Source: CAD feature listing. Evaluate the final solid. Frame: model axes, mm. A direction names the side the tool comes from. Coordinates: 2 decimals unless noted, no trailing zeros. Write each loop counter-clockwise with the first axis right and the second up, starting at its lowest first coordinate (ties: lowest second). Pieces come first, ordered by that corner, then holes. Notation, with made-up numbers: (11.5, -30) - (58.5, -30) arc R29 cw to (58.5, 6) - close; hole circle Ø3 at (76, 82). An arc over 180 degrees is marked (long way). One line per question, with ' | ' between items. Start each with the question number.
Q1. Line query: line 1 (Z direction, x = 76, y = 2.3); line 2 (Z direction, x = 76, y = 0.8); line 3 (X direction, y = 2.45, z = 30). Output: solid intervals per line, ascending.
Q2. Cut plane B-B, the plane x = 16. Return loops of the section in (y, z), plus the area to 3 significant figures.
Q3. Contact query for flat-ended pins moving along their axis: P1, Ø1.5, axis at y = 2, z = -9, coming from the +X side; P2, Ø4, axis at x = 76, z = -30, coming from the -Y side; P3, Ø0.9, axis at x = 91.5, y = 1, coming from the -Z side. Output: stop coordinate, or through.
Q4. Cut plane C-C, the plane x = -44. Return loops of the section in (y, z), plus the area to 3 significant figures.
Q5. Cut plane A-A, the plane z = 0. Return loops of the section in (x, y), plus the area to 3 significant figures.
Q6. Cut plane D-D, the plane y = 2.35. Give the number of separate pieces and of enclosed holes in the cut face, plus the area to 3 significant figures.
Q7. Access query for faces 5 (the face through (-58.8, 2, 20)), 6 (the face through (90.641, 1.479, 41.203)), 7 (the face through (96.07, 1.48, 53.5)). Directions: +Z, -Z, +X, -X, +Y, -Y. A direction counts if a zero-diameter tool reaches every point of the face in a straight line with its end or side. Return the directions, or none.
Q8. Draft query along X for faces 1 (the face through (52.95, 1.52, 15.32)), 2 (the face through (-65.5, 2, -27)), 3 (the face through (-44.208, 2.31, -31.586)), 4 (the face through (90.703, 1.479, 47.859)). Return one class per face: +X half, -X half, draft (parallel to the pull), parting line (faces both ways), or undercut.
Autodesk Inventor part; units mm, degrees
ref_plane "YZ Plane" through (0, 0, 0) normal (1, 0, 0) x (0, 1, 0)
ref_plane "XZ Plane" through (0, 0, 0) normal (0, 1, 0) x (-1, 0, 0)
ref_plane "XY Plane" through (0, 0, 0) normal (0, 0, 1) x (1, 0, 0)
sketch "Sketch1" plane through (0, 0, 0) normal (0, 1, 0) x (-1, 0, 0)
  circle A0 centre (0, 0) radius 40
  circle A1 centre (0, 0) radius 25
  dimension "d1" = 50
  dimension "d13" = 15
extrude "Extrusion1" add sketch "Sketch1" along normal blind 5
sketch "Sketch2" plane through (0, 5, 0) normal (0, 1, 0) x (1, 0, 0)
  circle A0 centre (-33, 0) radius 1.25
  circle A1 centre (0, 0) radius 25
  circle A2 centre (0, 0) radius 33 construction
  dimension "d4" = 2.5
  dimension "d12" = 8
extrude "Extrusion2" cut sketch "Sketch2" against normal blind 10 contours A0
pattern_circular "Circular Pattern1" count 6 over 360 about axis through (0, 0, 0) along (0, 1, 0) of "Extrusion2"
sketch "Sketch3" plane through (0, 5, 0) normal (0, 1, 0) x (1, 0, 0)
  line L0 (-85, -42.5) -> (85, -42.5)
  line L1 (85, -42.5) -> (85, 42.5)
  line L2 (85, 42.5) -> (-85, 42.5)
  line L3 (-85, 42.5) -> (-85, -42.5)
  line L4 (-85, -42.5) -> (85, 42.5) construction
  line L5 (85, -42.5) -> (-85, 42.5) construction
  line L6 (34.5, 15.5) -> (65.5, 15.5) construction
  line L7 (65.5, 15.5) -> (65.5, -15.5) construction
  line L8 (65.5, -15.5) -> (34.5, -15.5) construction
  line L9 (34.5, -15.5) -> (34.5, 15.5) construction
  line L10 (34.5, 15.5) -> (65.5, -15.5) construction
  line L11 (65.5, 15.5) -> (34.5, -15.5) construction
  circle A0 centre (34.5, 15.5) radius 1.5
  circle A1 centre (65.5, 15.5) radius 1.5
  circle A2 centre (65.5, -15.5) radius 1.5
  circle A3 centre (34.5, -15.5) radius 1.5
  line L12 (0, 0) -> (50, 0) construction
  circle A4 centre (0, 0) radius 40
  circle A5 centre (0, 0) radius 40
  line L13 (-50, 42.5) -> (-50, -42.5)
  circle A6 centre (50, 0) radius 12
  dimension "d14" = 85
  dimension "d15" = 170
  dimension "d16" = 31
  dimension "d17" = 31
  dimension "d18" = 3
  dimension "d19" = 3
  dimension "d20" = 3
  dimension "d21" = 3
  dimension "d22" = 50
  dimension "d23" = 35
  dimension "d26" = 24
extrude "Extrusion3" add sketch "Sketch3" against normal blind 5 contours L13 L2 L1 L0
sketch "Sketch4" plane through (0, 5, 0) normal (0, 1, 0) x (1, 0, 0)
  arc A0 (39.56, -5.9166) -> (39.56, 5.9166) centre (50, 0) ccw
  circle A1 centre (50, 0) radius 12
  point P0 (0, 0)
  point P1 (39.56, 5.9166)
  point P2 (39.56, -5.9166)
extrude "Extrusion4" cut sketch "Sketch4" against normal blind 5
sketch "Sketch5" plane through (0, 5, 0) normal (0, 1, 0) x (1, 0, 0)
  circle A0 centre (65.5, 15.5) radius 1.5
  circle A1 centre (65.5, 15.5) radius 1.5
  line L0 (34.5, -15.5) -> (65.5, -15.5)
  line L1 (65.5, -15.5) -> (65.5, 15.5)
  line L2 (65.5, 15.5) -> (34.5, 15.5)
  line L3 (34.5, 15.5) -> (34.5, -15.5)
  circle A2 centre (50, 0) radius 12
  line L4 (34.5, -15.5) -> (65.5, 15.5) construction
  line L5 (65.5, -15.5) -> (34.5, 15.5) construction
  circle A3 centre (34.5, 15.5) radius 1.5
  circle A4 centre (34.5, -15.5) radius 1.5
  point P0 (0, 0)
  dimension "d30" = 3
  dimension "d31" = 3
extrude "Extrusion5" cut sketch "Sketch5" against normal blind 5 contours A3 L3 L2 | L2 L3 A3 | A4 L3 L0 | L0 L3 A4
sketch "Sketch6" plane through (0, 5, 0) normal (0, 1, 0) x (1, 0, 0)
  line L0 (-65.5, -55) -> (97.5, -55)
  line L1 (97.5, -55) -> (97.5, 55)
  line L2 (97.5, 55) -> (-65.5, 55)
  line L3 (-65.5, 55) -> (-65.5, -55)
  line L4 (-65.5, -55) -> (97.5, 55) construction
  line L5 (97.5, -55) -> (-65.5, 55) construction
  line L6 (-65.5, 4) -> (-58.8, 4)
  line L7 (-58.8, 4) -> (-58.8, -55)
  line L8 (-58.8, -55) -> (-65.5, -55)
  line L9 (-65.5, -55) -> (-65.5, 4)
  line L10 (97.5, 55) -> (90.8, 55)
  line L11 (90.8, 55) -> (90.8, -4)
  line L12 (90.8, -4) -> (97.5, -4)
  line L13 (97.5, -4) -> (97.5, 55)
  line L14 (-50, -42.5) -> (-50, 42.5)
  line L15 (85, 42.5) -> (85, -42.5)
  line L16 (-50, 42.5) -> (85, 42.5)
  line L17 (85, 42.5) -> (85, -42.5)
  line L18 (85, -42.5) -> (-50, -42.5)
  line L19 (-50, -42.5) -> (-50, 42.5)
  point P0 (0, 0)
  point P1 (16, 0)
  dimension "d34" = 16
  dimension "d35" = 110
  dimension "d36" = 163
  dimension "d37" = 6.7
  dimension "d38" = 6.7
  dimension "d40" = 51
  dimension "d41" = 51
extrude "Extrusion6" add sketch "Sketch6" against normal blind 5 contours L7 L6 L3 L2 L11 L12 L1 L0
sketch "Sketch7" plane through (0, 5, 0) normal (0, 1, 0) x (1, 0, 0)
  line L0 (97.5, -49) -> (89.5, -49)
  line L1 (89.5, -49) -> (89.5, -40)
  line L2 (89.5, -40) -> (97.5, -40)
  line L3 (97.5, -40) -> (97.5, -49)
  line L4 (-58.8, -55) -> (97.5, -55)
  line L5 (97.5, -55) -> (97.5, -4)
  line L6 (97.5, -28) -> (93.5, -28)
  line L7 (93.5, -28) -> (93.5, -32)
  line L8 (93.5, -32) -> (97.5, -32)
  line L9 (97.5, -32) -> (97.5, -28)
  point P0 (0, 0)
  dimension "d44" = 6
  dimension "d45" = 9
  dimension "d46" = 8
  dimension "d47" = 8
  dimension "d48" = 4
  dimension "d49" = 4
extrude "Extrusion7" cut sketch "Sketch7" against normal blind 5
fillet "Fillet2" radius 2 2 edges at (97.5, 2.5, 28) (97.5, 2.5, 32)
fillet "Fillet3" radius 1 2 edges at (93.5, 2.5, 28) (93.5, 2.5, 32)
fillet "Fillet4" radius 1 2 edges at (97.5, 2.5, 49) (97.5, 2.5, 40)
fillet "Fillet5" radius 5 1 edges at (97.5, 2.5, 55)
fillet "Fillet6" radius 4 2 edges at (89.5, 2.5, 40) (89.5, 2.5, 49)
fillet "Fillet7" radius 5 2 edges at (97.5, 2.5, 4) (-65.5, 2.5, -4)
fillet "Fillet8" radius 10 3 edges at (-58.8, 2.5, 55) (90.8, 2.5, -55) (-65.5, 2.5, -55)
sketch "Sketch8" plane through (0, 5, 0) normal (0, 1, 0) x (1, 0, 0)
  circle A0 centre (-61.5, 8) radius 1.35
  circle A1 centre (93.5, -8) radius 1.35
  line L0 (-60.5, 4) -> (-58.8, 4)
  line L1 (-65.5, 45) -> (-65.5, 9)
  line L2 (92.5, -4) -> (90.8, -4)
  line L3 (97.5, -26) -> (97.5, -9)
  point P0 (0, 0)
  dimension "d59" = 4
  dimension "d60" = 4
  dimension "d61" = 2.7
  dimension "d62" = 4
  dimension "d63" = 4
  dimension "d64" = 2.7
extrude "Extrusion8" cut sketch "Sketch8" against normal blind 5
sketch "Sketch9" plane through (0, 5, 0) normal (0, 1, 0) x (1, 0, 0)
  line L0 (-48, 44) -> (76, 44)
  line L1 (76, 44) -> (76, -39)
  line L2 (76, -39) -> (-48, -39)
  line L3 (-48, -39) -> (-48, 44)
  point P0 (0, 0)
extrude "Extrusion9" add sketch "Sketch9" against normal blind 5
sketch "Sketch10" plane through (0, 5, 0) normal (0, 1, 0) x (1, 0, 0)
  circle A0 centre (16, 0) radius 40
  line L0 (-58.8, 4) -> (-58.8, -45)
  point P0 (0, 0)
  dimension "d69" = 80
  dimension "d70" = 74.8
extrude "Extrusion10" cut sketch "Sketch10" against normal blind 5
sketch "Sketch11" plane through (0, 5, 0) normal (0, 1, 0) x (1, 0, 0)
  line L0 (-44, -30) -> (76, -30) construction
  line L1 (76, -30) -> (76, 30) construction
  line L2 (76, 30) -> (-44, 30) construction
  line L3 (-44, 30) -> (-44, -30) construction
  circle A0 centre (16, 0) radius 40 construction
  line L4 (-44, -30) -> (76, 30) construction
  line L5 (76, -30) -> (-44, 30) construction
  circle A1 centre (76, 30) radius 1.6
  circle A2 centre (-44, 30) radius 1.6
  circle A3 centre (-44, -30) radius 1.6
  circle A4 centre (76, -30) radius 1.6
  point P0 (0, 0)
  dimension "d73" = 60
  dimension "d74" = 120
  dimension "d75" = 3.2
  dimension "d76" = 3.2
  dimension "d77" = 3.2
  dimension "d78" = 3.2
extrude "Extrusion11" cut sketch "Sketch11" against normal blind 5
sketch "Sketch12" plane through (0, 5, 0) normal (0, 1, 0) x (1, 0, 0)
  line L0 (-160, 70) -> (160, 70)
  line L1 (160, 70) -> (160, -70)
  line L2 (160, -70) -> (-160, -70)
  line L3 (-160, -70) -> (-160, 70)
  line L4 (-160, 70) -> (160, -70) construction
  line L5 (160, 70) -> (-160, -70) construction
  point P0 (0, 0)
extrude "Extrusion12" cut sketch "Sketch12" against normal blind 2
chamfer "Chamfer1" distance 1.6 angle 45 4 edges at (-45.6, 0, 30) (74.4, 0, 30) (74.4, 0, -30) (-45.6, 0, -30)
properties part number "Microscope lid"
Reply:
1) line 1: z = -55 to -31.6, -28.4 to 28.4, 31.6 to 55 | line 2: z = -55 to -32.4, -27.6 to 27.6, 32.4 to 55 | line 3: x = -58.8 to -45.6, -42.4 to -10.46, 42.46 to 74.4, 77.6 to 93.5
2) outline: (0, -55) - (3, -55) - (3, -40) - (0, -40) - close; (0, 40) - (3, 40) - (3, 55) - (0, 55) - close | area: 90.0 mm^2
3) P1: stops at x = 90.8 | P2: stops at y = 1.2 | P3: stops at z = 4
4) outline: (0, -55) - (3, -55) - (3, -31.6) - (1.6, -31.6) - (0, -33.2) - close; (0, -26.8) - (1.6, -28.4) - (3, -28.4) - (3, 28.4) - (1.6, 28.4) - (0, 26.8) - close; (0, 33.2) - (1.6, 31.6) - (3, 31.6) - (3, 55) - (0, 55) - close | area: 306 mm^2
5) outline: (-58.8, 0) - (-24, 0) - (-24, 3) - (-58.8, 3) - close; (56, 0) - (90.8, 0) - (90.8, 3) - (56, 3) - close | area: 209 mm^2
6) separate pieces: 1 | enclosed holes: 7 | area: 11,900 mm^2
7) face 5: +Z, -X, +Y, -Y | face 6: +X, +Y, -Y | face 7: +Z, +X, +Y, -Y
8) face 1: undercut | face 2: -X half | face 3: undercut | face 4: +X half
